from build123d import *

# Parameters (mm, degrees)
SKETCH1_W           = 122
SKETCH1_H           = 44
SKETCH1_R           = 2
BOSS_EXTRUDE1_DEPTH = 1.6
SKETCH2_W           = 106
SKETCH2_H           = 35.5
BOSS_EXTRUDE2_DEPTH = 8.5
SKETCH4_W           = 99
SKETCH4_H           = 24
CUT_EXTRUDE1_DEPTH  = 1
BOSS_EXTRUDE3_DEPTH = 3.4


with BuildPart() as part:
    # Sketch1 → Boss-Extrude1 (new body)
    with BuildSketch(Plane.XY):
        Rectangle(SKETCH1_W, SKETCH1_H)
        with Locations((-57.5, 18.5)):
            Circle(SKETCH1_R, mode=Mode.SUBTRACT)
        with Locations((-57.5, -18.5)):
            Circle(SKETCH1_R, mode=Mode.SUBTRACT)
        with Locations((57.5, 18.5)):
            Circle(SKETCH1_R, mode=Mode.SUBTRACT)
        with Locations((57.5, -18.5)):
            Circle(SKETCH1_R, mode=Mode.SUBTRACT)
    extrude(amount=BOSS_EXTRUDE1_DEPTH)

    # Sketch2 → Boss-Extrude2 (add)
    with BuildSketch(Plane.XY.offset(1.6)):
        with Locations((0, 2)):
            Rectangle(SKETCH2_W, SKETCH2_H)
    extrude(amount=BOSS_EXTRUDE2_DEPTH)

    # Sketch4 → Cut-Extrude1 (cut)
    with BuildSketch(Plane.XY.offset(10.1)):
        with Locations((0, 2)):
            Rectangle(SKETCH4_W, SKETCH4_H)
    extrude(amount=-CUT_EXTRUDE1_DEPTH, mode=Mode.SUBTRACT)

    # Sketch5 → Boss-Extrude3 (add)
    with BuildSketch(Plane.XY.offset(1.6)):
        Polygon((53, 15.75), (53, -11.75), (57.5, -8), (57.5, 12), align=None)
    extrude(amount=BOSS_EXTRUDE3_DEPTH)


solid = part.part
Can you work these out from the model? Positions are in its coordinate system, mm. A direction names the side the tool comes from. Coordinates: 2 decimals unless noted, no trailing zeros. Write each loop counter-clockwise with the first axis right and the second up, starting at its lowest first coordinate (ties: lowest second). Pieces come first, ordered by that corner, then holes. Notation, with made-up numbers: (26.5, 42.5) -> (71.5, 42.5) arc R21 ccw to (71.5, 54.5) -> close; hole circle Ø7 at (26.5, 37.25). An arc over 180 degrees is marked (long way). Write each question's results on one line, items separated by ' | '. Start each with the question number.
Item 1: I'm going to push flat-ended pins straight in: P1, Ø5, axis at x = -57.5, y = -18.5, coming from the +Z side; P2, Ø1.3, axis at x = 54.5, y = -0.5, coming from the +Z side; P3, Ø5, axis at x = 57.5, y = -18.5, coming from the -Z side; P4, Ø3, axis at y = 16.5, z = 3.5, coming from the -X side. Where does each tip first touch, or does it pass through?
Item 2: Please list where these lines run through material, in increasing order: probe 1 along Y at (x, z) = (57.5, 0.65); probe 2 along Y at (x, z) = (56.5, 0.75); probe 3 along Y at (x, z) = (-41.5, 2.5).
Item 3: If we section it at B-B, the plane x = -57.5: Write out the boundary of the cut face in (y, z), and give its area (3 significant figures).
Item 4: If we section it at C-C, the plane x = 1: Write out the boundary of the cut face in (y, z), and give its area (3 significant figures).
Item 5: If we section it at D-D, the plane y = -13.5: Write out the boundary of the cut face in (x, z).
Item 6: Thinking about a two-plate mould opening in Y: for faces 1 (the flat face through (-53, 2, 6)), 2 (the flat face through (-1, -15.75, 6)), 3 (the cylindrical face through (58.575, -16.814, 0.789)), 4 (the cylindrical face through (59.408, 19.101, 0.789)), which applies, released by +Y, released by -Y, zero draft, split by the parting line, or undercut?
Item 7: On a 3-axis mill with a long thin cutter (end or side, diameter ignored), from which of +Z, -Z, +X, -X, +Y, -Y can I reach the whole of each face in a straight line? I mean faces 5 (the flat face through (-1, 19.75, 6)), 6 (the flat face through (55, 2, 5)), 7 (the flat face through (55.22, -9.9, 3.28)), 8 (the flat face through (55.28, 13.85, 3.28)), 9 (the flat face through (-1, 2, 9.1)). Say none if no direction works.
Item 8: If we section it at A-A, the plane y = 18.5: Write out the boundary of the cut face in (x, z).
Answer block:
1) P1: z = 1.6 | P2: z = 5 | P3: z = 0 | P4: x = -53
2) probe 1: -22 to -20.5, -16.5 to 16.5, 20.5 to 22 | probe 2: -22 to -20.23, -16.77 to 16.77, 20.23 to 22 | probe 3: -15.75 to 19.75
3) outline: (-22, 0) -> (-20.5, 0) -> (-20.5, 1.6) -> (-22, 1.6) -> close; (-16.5, 0) -> (16.5, 0) -> (16.5, 1.6) -> (-16.5, 1.6) -> close; (20.5, 0) -> (22, 0) -> (22, 1.6) -> (20.5, 1.6) -> close | area: 57.6 mm²
4) outline: (-22, 0) -> (22, 0) -> (22, 1.6) -> (19.75, 1.6) -> (19.75, 10.1) -> (14, 10.1) -> (14, 9.1) -> (-10, 9.1) -> (-10, 10.1) -> (-15.75, 10.1) -> (-15.75, 1.6) -> (-22, 1.6) -> close | area: 348 mm²
5) outline: (-61, 0) -> (61, 0) -> (61, 1.6) -> (53, 1.6) -> (53, 10.1) -> (-53, 10.1) -> (-53, 1.6) -> (-61, 1.6) -> close
6) face 1: zero draft | face 2: released by -Y | face 3: undercut | face 4: undercut
7) face 5: +Z, +X, -X, +Y | face 6: +Z, +X, +Y, -Y | face 7: +Z, +X, -Y | face 8: +Z, +X, +Y | face 9: +Z
8) outline: (-61, 0) -> (-59.5, 0) -> (-59.5, 1.6) -> (-61, 1.6) -> close; (-55.5, 0) -> (55.5, 0) -> (55.5, 1.6) -> (53, 1.6) -> (53, 10.1) -> (-53, 10.1) -> (-53, 1.6) -> (-55.5, 1.6) -> close; (59.5, 0) -> (61, 0) -> (61, 1.6) -> (59.5, 1.6) -> close
